Geometry: see drawing. Coordinates: mm, zero at the bounding-box minimum. A direction names the side the tool comes from. Give positions to 0.01 mm unless a question says otherwise; leave off trailing zeros. Write each loop counter-clockwise with the first axis right and the second up, starting at its lowest first coordinate (ties: lowest second). Pieces come first, ordered by that corner, then holes.
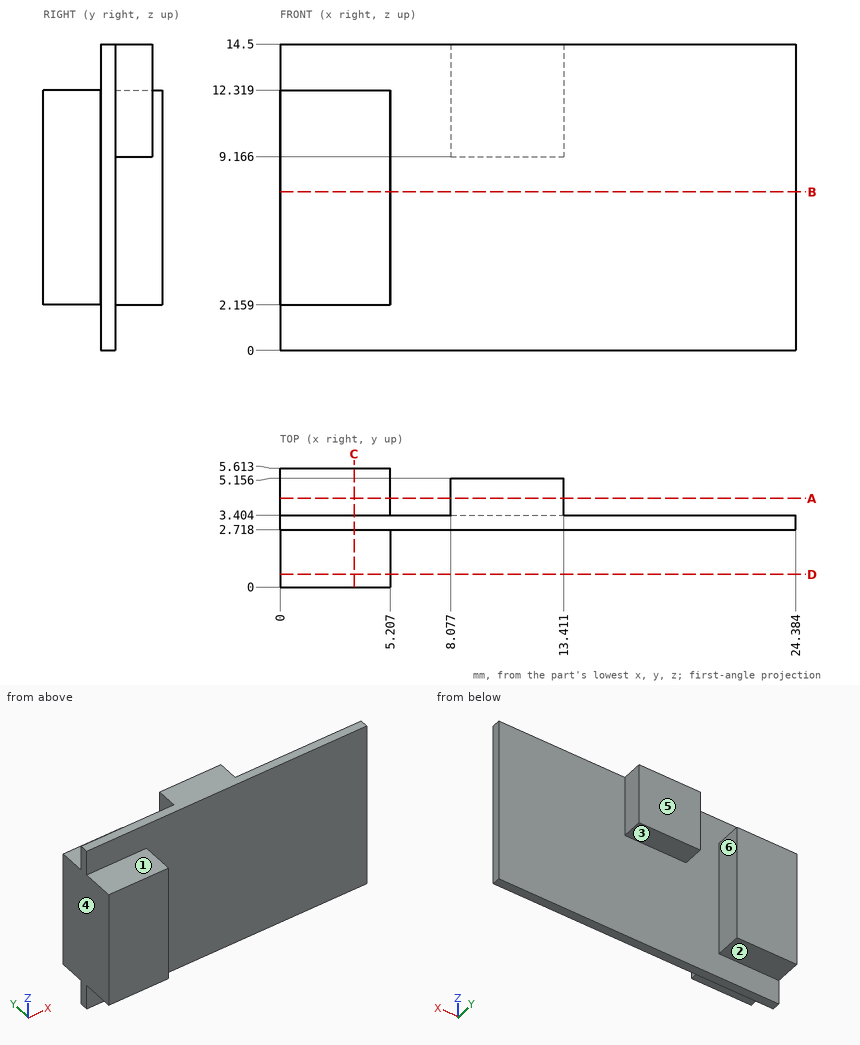
Q1. Section A-A, the plane y = 4.2. Return the cut outline in (x, z).
Q2. Mould query, pull axis X, two halves, no side actions, for the marked faces 4, 5 and 6. Classes: +X half, -X half, draft (parallel to the pull), parting line (faces both ways), or undercut.
Q3. Section C-C, the plane x = 3.5. Return the cut outline in (y, z), then the cut area to 3 significant figures.
Q4. Section B-B, the plane z = 7.5. Return the cut outline in (x, y).
Q5. Section D-D, the plane y = 0.6. Return the cut outline in (x, z).
Q6. Access query for the marked faces 1, 2 and 3. Directions: +Z, -Z, +X, -X, +Y, -Y. A direction counts if a zero-diameter tool reaches every point of the face in a straight line with its end or side. Return the directions, or none.
Q7. Material intervals for line 1 along X through (y, z) = (1.85, 3.5); line 2 along Z through (x, y) = (2.5, 2.2); line 3 along Y through (x, z) = (13.75, 6), sorted ascending.
Q8. Pin query (flat end, axial travel): pin 1 (2 mm diameter, centred on y = 2, z = 5.5, fed in from +X); pin 2 (1.4 mm diameter, centred on x = 2, y = 1, fed in from +Z); pin 3 (2 mm diameter, centred on x = 15.5, z = 13, fed in from -Y); pin 4 (0.7 mm diameter, centred on x = 1.5, y = 4, fed in from -Z). Return the tip coordinate at first contact, or that it passes through.
Solutions:
1. outline: (0, 2.16) - (5.21, 2.16) - (5.21, 12.32) - (0, 12.32) - close; (8.08, 9.17) - (13.41, 9.17) - (13.41, 14.5) - (8.08, 14.5) - close
2. face 4: -X half
2. face 5: draft
2. face 6: undercut
3. outline: (0, 2.16) - (2.72, 2.16) - (2.72, 0) - (3.4, 0) - (3.4, 2.16) - (5.61, 2.16) - (5.61, 12.32) - (3.4, 12.32) - (3.4, 14.5) - (2.72, 14.5) - (2.72, 12.32) - (0, 12.32) - close
3. area: 60.0 mm2
4. outline: (0, 0) - (5.21, 0) - (5.21, 2.72) - (24.38, 2.72) - (24.38, 3.4) - (5.21, 3.4) - (5.21, 5.61) - (0, 5.61) - close
5. outline: (0, 2.16) - (5.21, 2.16) - (5.21, 12.32) - (0, 12.32) - close
6. face 1: +Z, +X, -X, -Y
6. face 2: -Z, +X, -X, +Y
6. face 3: -Z, +X, +Y
7. line 1: x = 0 to 5.21
7. line 2: z = 2.16 to 12.32
7. line 3: y = 2.72 to 3.4
8. pin 1: stops at x = 24.38
8. pin 2: stops at z = 12.32
8. pin 3: stops at y = 2.72
8. pin 4: stops at z = 2.16
